```python
from build123d import *

# Parameters (mm, degrees)
F1_DEPTH = 39
F2_R     = 2.5
F3_DEPTH = 2.748386896
F4_R     = 4.1378331658
F4_R_2   = 4.1919705303
F5_DEPTH = 27.748386896
F6_W     = 71.9977971367
F6_H     = 25
F7_DEPTH = 5
F8_W     = 71.9977971367
F8_H     = 27.748386896
F9_DEPTH = 5


with BuildPart() as f1:
    # F0 (on Front) → F1 (new body, symmetric)
    with BuildSketch(Plane.XZ):
        Polygon((33.0240737289, -6.6249261405), (-2.9748248395, -6.6249261405), (-2.9748248395, -9.6249261405), (36.0251751605, -9.6249261405), (36.0251751605, 18.3750738595), (48.0240737289, 18.3750738595), (48.0240737289, 21.1234607555), (33.0240737289, 21.1234607555), align=None)
        Polygon((-2.9748248395, -9.6249261405), (-2.9748248395, -6.6249261405), (-38.9737234078, -6.6249261405), (-38.9737234078, 21.1234607555), (-53.9737234078, 21.1234607555), (-53.9737234078, 18.3750738595), (-41.9748248395, 18.3750738595), (-41.9748248395, -9.6249261405), align=None)
    extrude(amount=F1_DEPTH, both=True)

    # F2 (on face) → F3 (cut, through all)
    with BuildSketch(Plane.XY.offset(21.1234607555)):
        with Locations((42.0246244447, -24)):
            Circle(F2_R)
        with Locations((42.0246244447, 24)):
            Circle(F2_R)
        with Locations((-47.9742741236, 24)):
            Circle(F2_R)
        with Locations((-47.9742741236, -24)):
            Circle(F2_R)
    extrude(amount=-F3_DEPTH, mode=Mode.SUBTRACT)

    # F4 (on face) → F5 (join, through all)
    with BuildSketch(Plane.XY.offset(-6.6249261405)):
        with Locations((15.3820728883, 24.0051727742)):
            Circle(F4_R)
        with Locations((15.3820728883, -24.139655754)):
            Circle(F4_R)
        with Locations((-19.8524110019, 24.139655754)):
            Circle(F4_R)
        with Locations((-19.4489639252, -24.2741387337)):
            Circle(F4_R_2)
    extrude(amount=F5_DEPTH)

    # F6 (on face) → F7 (join)
    with BuildSketch(Plane.XZ.offset(39)):
        with Locations((-2.9748248395, 5.8750738595)):
            Rectangle(F6_W, F6_H)
    extrude(amount=-F7_DEPTH)

    # F8 (on face) → F9 (join)
    with BuildSketch(Plane(origin=(0, 39, 0), x_dir=(-1, 0, 0), z_dir=(0, 1, 0))):
        with Locations((2.9748248395, 7.2492673075)):
            Rectangle(F8_W, F8_H)
    extrude(amount=-F9_DEPTH)


solid = f1.part
```
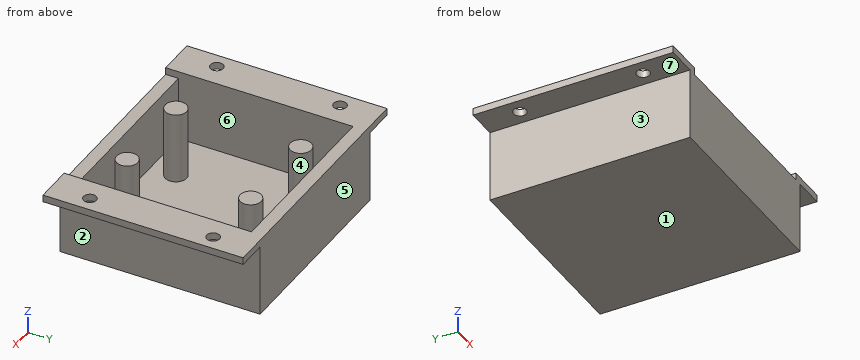
Read the model definition and answer for the solid it produces. Units are mm, in the model's axes. Face numbers are marked on the shaded views. A direction names the side the tool comes from. Give positions to 0.01 mm unless a question says otherwise; leave off trailing zeros. Order: outer loops, then holes, each group sorted by start corner. A loop starts at its lowest first (then second) coordinate and runs counter-clockwise, first axis right, second up. Notation, with made-up numbers: (10.25, 37) -> (65.25, 37) arc R32 cw to (65.25, 72) -> close; hole circle Ø1 at (64, -9.75). An arc over 180 degrees is marked (long way). One line per item, written item: value. Start each with the question number.
(1) For a pull along Y with two mould halves and no side action, classify the marked faces 5, 6 and 7 as released by +Y, released by -Y, zero draft, split by the parting line, or undercut.
(2) The part is cut by section A-A (z = -4). Determine the outline of the cut face in (x, y).
(3) Straight lines are drawn through the part: L1, parallel to X at y = 12.5, z = 16; L2, parallel to Y at x = 10.5, z = 13.5; L3, parallel to X at y = 24, z = 4.5. For each, find the intervals that lie inside material, in ascending order.
(4) The part is cut by section C-C (y = 15). Determine the outline of the cut face in (x, z).
(5) Flat-ended cylindrical pins translate along their axes: P1, Ø5, axis at y = 0, z = 14.5, coming from the +X side; P2, Ø3.5, axis at x = -48, y = -6.5, coming from the -Z side; P3, Ø4, axis at x = -47.97, y = -24, coming from the +Z side; P4, Ø8, axis at x = -8, y = 3, coming from the +Z side. Find the tip coordinate at first contact, or state that the pin passes through.
(6) The part is cut by section D-D (x = -21). Determine the outline of the cut face in (y, z), and give its area (4 significant figures).
(7) The part is cut by section B-B (x = 0.5). Determine the outline of the cut face in (y, z).
(8) A tool of negligible diameter and unlimited length cuts with its end or side. For the marked faces 1, 2, 3 and 4, from which of +Z, -Z, +X, -X, +Y, -Y can it reach the whole face along a straight path? Write none if from no direction.
Taken from the geometry:
1. face 5: released by +Y
1. face 6: undercut
1. face 7: zero draft
2. outline: (-41.97, -39) -> (36.03, -39) -> (36.03, 39) -> (-41.97, 39) -> close; circle Ø8.28 at (-19.85, 24.14); circle Ø8.38 at (-19.45, -24.27); circle Ø8.28 at (15.38, -24.14); circle Ø8.28 at (15.38, 24.01); hole (-38.97, -34) -> (33.02, -34) -> (33.02, 34) -> (-38.97, 34) -> close
3. L1: -41.97 to -38.97, 33.02 to 36.03
3. L2: -39 to -34, 34 to 39
3. L3: -41.97 to -38.97, -23.99 to -15.72, 11.24 to 19.52, 33.02 to 36.03
4. outline: (-53.97, 18.38) -> (-41.97, 18.38) -> (-41.97, -9.62) -> (36.03, -9.62) -> (36.03, 18.38) -> (48.02, 18.38) -> (48.02, 21.12) -> (33.02, 21.12) -> (33.02, -6.62) -> (-38.97, -6.62) -> (-38.97, 21.12) -> (-53.97, 21.12) -> close
5. P1: x = 36.03
5. P2: z = 18.38
5. P3: through
5. P4: z = -6.62
6. outline: (-39, -9.62) -> (39, -9.62) -> (39, 21.12) -> (34, 21.12) -> (34, -6.62) -> (28.12, -6.62) -> (28.12, 21.12) -> (20.16, 21.12) -> (20.16, -6.62) -> (-20.38, -6.62) -> (-20.38, 21.12) -> (-28.17, 21.12) -> (-28.17, -6.62) -> (-34, -6.62) -> (-34, 18.38) -> (-39, 18.38) -> close
6. area: 934.5 mm^2
7. outline: (-39, -9.62) -> (39, -9.62) -> (39, 21.12) -> (34, 21.12) -> (34, -6.62) -> (-34, -6.62) -> (-34, 18.38) -> (-39, 18.38) -> close
8. face 1: -Z, +X, -X, +Y, -Y
8. face 2: -Z, +X, +Y, -Y
8. face 3: -Z, -X, +Y, -Y
8. face 4: +Z
